For this review, use the dimensioned drawing (mm, ordinates from the lowest corner) and the shaded views. A direction names the side the tool comes from. Give positions to 0.01 mm unless a question says otherwise; leave off trailing zeros. Order: outer loops, then holes, each group sorted by start corner. A loop starts at its lowest first (then second) coordinate and runs counter-clockwise, first axis right, second up. Notation, with made-up numbers: (65, 42.25) - (96, 42.25) arc R34 ccw to (96, 73.25) - close; hole circle Ø2 at (-24, 34). An arc over 180 degrees is marked (long way). Use a Markdown table: item, result. Add a question column.
1) Mouldability with a two-part tool opening along X and no side actions: class the marked faces 1, 2 and 3 as released by +X, released by -X, zero draft, split by the parting line, or undercut.
2) We need section C-C on z = 1.25. Write out the cut boundary in (x, y), then the cut area to 3 significant figures.
3) Machinability: for the marked faces 4 and 5, which of the approach directions +Z, -Z, +X, -X, +Y, -Y give a long, thin tool a straight path to every point of the face, cutting with its end or side? Answer none if there is none.
4) We need section A-A on z = 5. Write out the cut boundary in (x, y), then the cut area to 3 significant figures.
5) Clearance check with flat-ended pins moving along their axes: P1, Ø1.5, axis at y = 6, z = 7.5, coming from the -X side; P2, Ø1, axis at y = 9.5, z = 7.5, coming from the +X side; P3, Ø5, axis at x = 44.5, z = 6, coming from the +Y side. State where each tip first meets the part, or that it passes through.
6) We need section B-B on x = 45. Write out the cut boundary in (y, z), then the cut area to 3 significant figures.
7) We need section D-D on y = 7.75. Write out the cut boundary in (x, z).
8) Wall thickness on L1, parallel to X at y = 3.2, z = 5; L2, parallel to Z at x = 45, y = 3.1; L3, parallel to Y at x = 34.5, z = 4.5: over which ranges is each line inside the solid? List them lowest first.
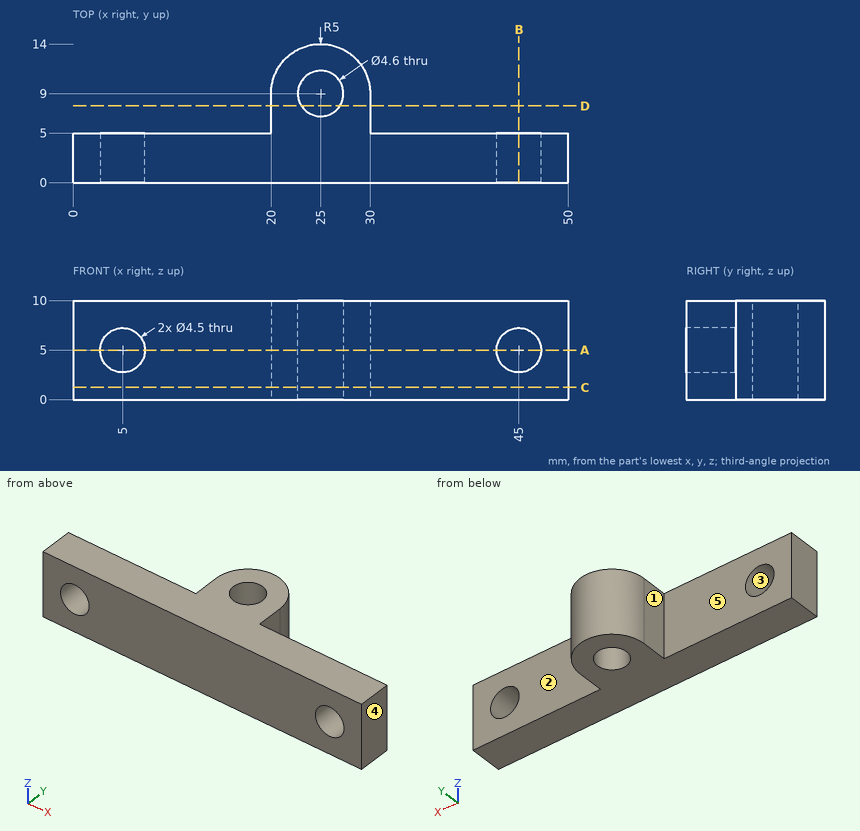
Checked values:
| question | item | result |
|---|---|---|
| 1 | face 1 | released by -X |
| 1 | face 2 | zero draft |
| 1 | face 3 | undercut |
| 2 | outline | (0, 0) - (50, 0) - (50, 5) - (30, 5) - (30, 9) arc R5 ccw to (20, 9) - (20, 5) - (0, 5) - close; hole circle Ø4.6 at (25, 9) |
| 2 | area | 313 mm² |
| 3 | face 4 | +Z, -Z, +X, +Y, -Y |
| 3 | face 5 | +Z, -Z, -X, +Y |
| 4 | outline | (0, 0) - (2.75, 0) - (2.75, 5) - (0, 5) - close; (7.25, 0) - (42.75, 0) - (42.75, 5) - (30, 5) - (30, 9) arc R5 ccw to (20, 9) - (20, 5) - (7.25, 5) - close; (47.25, 0) - (50, 0) - (50, 5) - (47.25, 5) - close; hole circle Ø4.6 at (25, 9) |
| 4 | area | 268 mm² |
| 5 | P1 | x = 20 |
| 5 | P2 | x = 30 |
| 5 | P3 | y = 5 |
| 6 | outline | (0, 0) - (5, 0) - (5, 2.75) - (0, 2.75) - close; (0, 7.25) - (5, 7.25) - (5, 10) - (0, 10) - close |
| 6 | area | 27.5 mm² |
| 7 | outline | (20, 0) - (23.07, 0) - (23.07, 10) - (20, 10) - close; (26.93, 0) - (30, 0) - (30, 10) - (26.93, 10) - close |
| 8 | L1 | 0 to 2.75, 7.25 to 42.75, 47.25 to 50 |
| 8 | L2 | 0 to 2.75, 7.25 to 10 |
| 8 | L3 | 0 to 5 |
